Build history of the part. All positions in model axes, mm. A direction names the side the tool comes from. Give positions to 0.01 mm unless a question says otherwise; leave off trailing zeros. Order: outer loops, then holes, each group sorted by start corner. A loop starts at its lowest first (then second) coordinate and runs counter-clockwise, first axis right, second up. Notation, with made-up numbers: (3, 22) - (62, 22) arc R22 ccw to (62, 30) - close; hole circle Ø8 at (68, 75.25). An arc over 180 degrees is marked (long way). Use a Markdown table: item, result.
from build123d import *

# Parameters (mm, degrees)
SKETCH1_R           = 2.5
BOSS_EXTRUDE1_DEPTH = 34
SKETCH2_R           = 1
CUT_EXTRUDE1_DEPTH  = 20
FILLET1_R           = 0.25


with BuildPart() as part:
    # Sketch1 → Boss-Extrude1 (new body, symmetric)
    with BuildSketch(Plane.XY):
        Circle(SKETCH1_R)
    extrude(amount=BOSS_EXTRUDE1_DEPTH, both=True)

    # Sketch2 → Cut-Extrude1 (cut)
    with BuildSketch(Plane.XY.offset(34)):
        Circle(SKETCH2_R)
    extrude(amount=-CUT_EXTRUDE1_DEPTH, mode=Mode.SUBTRACT)

    # Fillet1
    fillet1_edges = [part.edges().sort_by_distance(p)[0] for p in [
        (-2.5, 0, 34),
        (-1, 0, 34),
    ]]
    fillet(fillet1_edges, radius=FILLET1_R)


solid = part.part
1) Two-plate mould, pull along X, no slides. Class faces 3 (the cylindrical face through (-0.54, -2.44, 0.35)), 4 (the flat face through (1, -1, 34)), 5 (the cylindrical face through (0, -1, 24)): +X half, -X half, draft (parallel to the pull), parting line (faces both ways), or undercut.
Computed:
| item | result |
|---|---|
| face 3 | parting line |
| face 4 | draft |
| face 5 | undercut |
2) Slice it at A-A (x = 0). Write the cut outline in (y, z).
Computed:
| item | result |
|---|---|
| outline | (-2.5, -34) - (2.5, -34) - (2.5, 33.75) arc R0.25 ccw to (2.25, 34) - (1.25, 34) arc R0.25 ccw to (1, 33.75) - (1, 14) - (-1, 14) - (-1, 33.75) arc R0.25 ccw to (-1.25, 34) - (-2.25, 34) arc R0.25 ccw to (-2.5, 33.75) - close |
3) Wall check: line 1 (Y direction, x = 0, z = 29.5); line 2 (Z direction, x = 0.15, y = -0.85); line 3 (X direction, y = 0.35, z = 27.5). Give the ranges that are in metal, low to high. Write a range as from..to.
Computed:
| item | result |
|---|---|
| line 1 | y = -2.5..-1, 1..2.5 |
| line 2 | z = -34..14 |
| line 3 | x = -2.48..-0.94, 0.94..2.48 |
4) Tool access for faces 1 (the flat face through (0, 0, -34)), 2 (the flat face through (0, 0, 14)): list every direction of +Z, -Z, +X, -X, +Y, -Y with a clear straight run to the whole face (end or side of a thin tool).
Computed:
| item | result |
|---|---|
| face 1 | -Z, +X, -X, +Y, -Y |
| face 2 | +Z |
5) Pin check, flat tip, straight feed: P1, Ø1, axis at x = 0.5, y = 0.5, coming from the +Z side. Stop position of the tip, or through.
Computed:
| item | result |
|---|---|
| P1 | stops at z = 34 |
6) Slice it at B-B (z = 24.5). Write the cut outline in (x, y), and give its area (3 significant figures).
Computed:
| item | result |
|---|---|
| outline | circle Ø5 at (0, 0); hole circle Ø2 at (0, 0) |
| area | 16.5 mm² |
7) Slice it at D-D (z = -27.5). Write the cut outline in (x, y), and give its area (3 significant figures).
Computed:
| item | result |
|---|---|
| outline | circle Ø5 at (0, 0) |
| area | 19.6 mm² |
